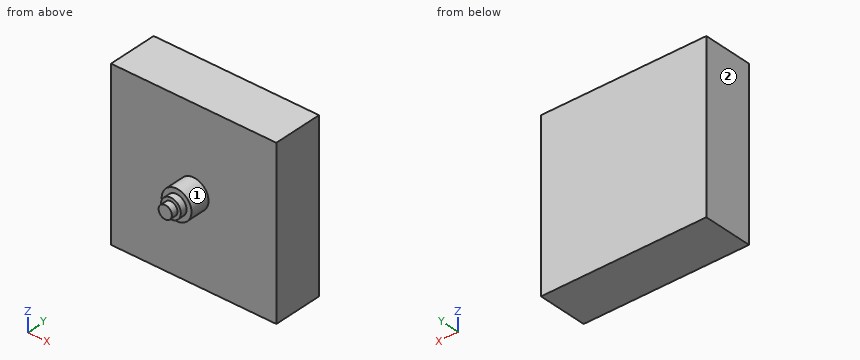
from build123d import *

# Parameters (mm, degrees)
F0_W     = 50
F0_H     = 50
F1_DEPTH = 15
F2_R     = 4.5
F3_DEPTH = 10
F4_R     = 4.5
F4_R_2   = 3
F5_DEPTH = 4
F6_R     = 3
F6_R_2   = 2
F7_DEPTH = 2


with BuildPart() as f1:
    # F0 (on Front) → F1 (new body)
    with BuildSketch(Plane.XZ):
        with Locations((25, 25)):
            Rectangle(F0_W, F0_H)
    extrude(amount=F1_DEPTH)

    # F2 (on face) → F3 (join)
    with BuildSketch(Plane.XZ.offset(15)):
        with Locations((25, 25)):
            Circle(F2_R)
    extrude(amount=F3_DEPTH)

    # F4 (on face) → F5 (cut)
    with BuildSketch(Plane.XZ.offset(25)):
        with Locations((25, 25)):
            Circle(F4_R)
        with Locations((25, 25)):
            Circle(F4_R_2, mode=Mode.SUBTRACT)
    extrude(amount=-F5_DEPTH, mode=Mode.SUBTRACT)

    # F6 (on face) → F7 (cut)
    with BuildSketch(Plane.XZ.offset(25)):
        with Locations((25, 25)):
            Circle(F6_R)
        with Locations((25, 25)):
            Circle(F6_R_2, mode=Mode.SUBTRACT)
    extrude(amount=-F7_DEPTH, mode=Mode.SUBTRACT)


solid = f1.part
Work out the finished part from the listing and answer in its coordinate system (mm). Face numbers are marked on the shaded views. A direction names the side the tool comes from. Give positions to 0.01 mm unless a question says otherwise; leave off trailing zeros. Write each loop counter-clockwise with the first axis right and the second up, starting at its lowest first coordinate (ties: lowest second). Pieces come first, ordered by that corner, then holes. Notation, with made-up numbers: (4.25, 82.5) - (15.25, 82.5) arc R31 ccw to (15.25, 106.5) - close; hole circle Ø7 at (26.25, -20). An arc over 180 degrees is marked (long way). One line per item, written item: value. Start each with the question number.
1. Consider probe 1 along Y at (x, z) = (29, 17); probe 2 along Y at (x, z) = (29, 25); probe 3 along X at (y, z) = (-15.5, 25.5). Determine where each line is inside the solid, lowest interval first.
2. Find section D-D (z = 32.5). Write down the section's boundary in (x, y).
3. For the marked faces 1 and 2, determine the directions among +Z, -Z, +X, -X, +Y, -Y from which every point of the face is accessible in a straight line to the end or side of a thin tool.
4. Find section B-B (z = 25). Write down the section's boundary in (x, y), then the cut area to 3 significant figures.
5. Find section C-C (y = -16.5). Write down the section's boundary in (x, z).
6. Given pin 1 (5 mm diameter, centred on x = 21.5, y = -21.5, fed in from -Z); pin 2 (2 mm diameter, centred on x = 10, z = 18.5, fed in from -Y), each flat-ended and moving along its own axis, determine where each tip first touches the part or whether it passes through.
7. Find section A-A (x = 25). Write down the section's boundary in (y, z), then the cut area to 3 significant figures.
Geometry results:
1. probe 1: -15 to 0
1. probe 2: -21 to 0
1. probe 3: 20.53 to 29.47
2. outline: (0, -15) - (50, -15) - (50, 0) - (0, 0) - close
3. face 1: -Y
3. face 2: +Z, -Z, -X, +Y, -Y
4. outline: (0, -15) - (20.5, -15) - (20.5, -21) - (22, -21) - (22, -23) - (23, -23) - (23, -25) - (27, -25) - (27, -23) - (28, -23) - (28, -21) - (29.5, -21) - (29.5, -15) - (50, -15) - (50, 0) - (0, 0) - close
4. area: 824 mm2
5. outline: circle Ø9 at (25, 25)
6. pin 1: z = 20.62
6. pin 2: y = -15
7. outline: (-25, 23) - (-23, 23) - (-23, 22) - (-21, 22) - (-21, 20.5) - (-15, 20.5) - (-15, 0) - (0, 0) - (0, 50) - (-15, 50) - (-15, 29.5) - (-21, 29.5) - (-21, 28) - (-23, 28) - (-23, 27) - (-25, 27) - close
7. area: 824 mm2
